from build123d import *

# Parameters (mm, degrees)
SKETCH1_R               = 1.5
BOSS_EXTRUDE1_DEPTH     = 5
EXTRUDE_THIN1_START     = -2.25
EXTRUDE_THIN1_OUTLINE_W = 10
EXTRUDE_THIN1_OUTLINE_H = 1
EXTRUDE_THIN1_DEPTH     = 4.5


# Read off the part's stored shape, not the designer's step: Extrude-Thin1
with BuildPart() as part:
    # Sketch1 → Boss-Extrude1 (new, symmetric)
    with BuildSketch(Plane(origin=(0, 0, 0), x_dir=(1, 0, 0), z_dir=(0, 1, 0))):
        with BuildLine():
            ThreePointArc((-14, 5), (-13.121320344, 7.121320344), (-11, 8))
            Line((-11, 8), (14, 8))
            Line((14, 8), (14, -5))
            ThreePointArc((14, -5), (13.121320344, -7.121320344), (11, -8))
            Line((11, -8), (-14, -8))
            Line((-14, -8), (-14, 5))
        make_face()
        with Locations(Location((-11.25, -5.5, 0), (0, 0, 270))):
            Circle(SKETCH1_R, mode=Mode.SUBTRACT)
        with Locations(Location((11, 5, 0), (0, 0, 270))):
            Circle(SKETCH1_R, mode=Mode.SUBTRACT)
    extrude(amount=BOSS_EXTRUDE1_DEPTH, both=True)

    # Extrude-Thin1 outline → Extrude-Thin1 (add)
    with BuildSketch(Plane(origin=(0, 0, 0), x_dir=(1, 0, 0), z_dir=(0, 1, 0)).offset(EXTRUDE_THIN1_START)):
        with Locations((19, -3.25)):
            Rectangle(EXTRUDE_THIN1_OUTLINE_W, EXTRUDE_THIN1_OUTLINE_H)
        with BuildLine():
            Line((1.5, 9.10197349), (1.5, 8))
            Line((1.5, 8), (2.5, 8))
            Line((2.5, 8), (2.5, 9.10197349))
            ThreePointArc((2.5, 9.10197349), (2.244023809, 9.770126595), (1.607142857, 10.096217126))
            Line((1.607142857, 10.096217126), (-25.338821814, 13))
            Line((-25.338821814, 13), (-25.445964671, 12.005756364))
            Line((-25.445964671, 12.005756364), (1.5, 9.10197349))
        make_face()
        with BuildLine():
            Line((1.3, -11), (10.3, -11))
            Line((10.3, -11), (10.3, -10))
            Line((10.3, -10), (1.3, -10))
            ThreePointArc((1.3, -10), (0.592893219, -9.707106781), (0.3, -9))
            Line((0.3, -9), (0.3, -8))
            Line((0.3, -8), (-0.7, -8))
            Line((-0.7, -8), (-0.7, -9))
            ThreePointArc((-0.7, -9), (-0.114213562, -10.414213562), (1.3, -11))
        make_face()
    extrude(amount=EXTRUDE_THIN1_DEPTH)


solid = part.part
Can you work these out from the model? Positions are in its coordinate system, mm. A direction names the side the tool comes from. Coordinates: 2 decimals unless noted, no trailing zeros. Order: outer loops, then holes, each group sorted by start corner. A loop starts at its lowest first (then second) coordinate and runs counter-clockwise, first axis right, second up. Notation, with made-up numbers: (48, 74.5) - (90, 74.5) arc R32 ccw to (90, 105.5) - close; hole circle Ø1 at (85, 62.25). An arc over 180 degrees is marked (long way). Answer as a JSON object with one key per item and string values. Group by question number.
Q1. On a 3-axis mill with a long thin cutter (end or side, diameter ignored), from which of +Z, -Z, +X, -X, +Y, -Y can I reach the whole of each face in a straight line? I mean faces 4 (the face through (3.5, -2.25, 10.15)), 5 (the face through (-12.162, -0.031, -10.574)), 6 (the face through (3.5, 2.25, 10.15)). Say none if no direction works.
Q2. We'd pull the mould along Z, two halves only. Please class faces 1 (the face through (-0.7, 0, 8.5)), 2 (the face through (1, 0, -8)), 3 (the face through (19, 0, 3.75)): +Z half, -Z half, draft (parallel to the pull), parting line (faces both ways), or undercut.
Q3. Imagine slicing it at B-B (z = 5.5). Please give me the cut outline in (x, y).
Q4. Imagine slicing it at A-A (y = -4). Please give me the cut outline in (x, z).
Q5. Imagine slicing it at D-D (z = 0.25). Please give me the cut outline in (x, y), and give its area (3 significant figures).
Q6. Will these pins go through, and if not, where does the flat tip stop? P1, Ø4, axis at x = -18, z = -11.5, coming from the +Y side; P2, Ø5, axis at y = -2.5, z = -6, coming from the -X side; P3, Ø2, axis at x = -19, z = -10.5, coming from the -Y side; P4, Ø0.9, axis at x = 7.5, z = 9, coming from the +Y side.
Q7. Imagine slicing it at C-C (x = 15). Please give me the cut outline in (y, z), and give its area (3 significant figures).
Q8. I need wall thicknesses on line 1 (X direction, y = -1, z = -5); line 2 (Z direction, x = 5, y = -3.25); line 3 (Z direction, x = -1, y = -1.75). Which ranges of each line are inside material? Lowest first, please. Write a range as from..to.
Determined:
{
 "1": {"face 4": "+Z, +X, -X, -Y", "face 5": "-X, +Y, -Y", "face 6": "+Z, +X, -X, +Y"},
 "2": {"face 1": "draft", "face 2": "undercut", "face 3": "+Z half"},
 "3": {"outline": "(-14, -5) - (-12.75, -5) - (-12.75, 5) - (-14, 5) - close; (-9.75, -5) - (13.96, -5) - (13.96, 5) - (-9.75, 5) - close"},
 "4": {"outline": "(-14, -5) arc R3 ccw to (-11, -8) - (14, -8) - (14, 5) arc R3 ccw to (11, 8) - (-14, 8) - close; hole circle Ø3 at (-11.25, 5.5); hole circle Ø3 at (11, -5)"},
 "5": {"outline": "(-14, -5) - (14, -5) - (14, 5) - (-14, 5) - close", "area": "280 mm2"},
 "6": {"P1": "stops at y = 2.25", "P2": "stops at x = -14", "P3": "stops at y = -2.25", "P4": "passes through"},
 "7": {"outline": "(-2.25, 2.75) - (2.25, 2.75) - (2.25, 3.75) - (-2.25, 3.75) - close", "area": "4.50 mm2"},
 "8": {"line 1": "x = -14..9.5, 12.5..14", "line 2": "z = -8..8", "line 3": "z = -10.38..-9.37, -8..8"}
}
